Autodesk Inventor part; units mm, degrees
ref_plane "YZ Plane" through (0, 0, 0) normal (1, 0, 0) x (0, 1, 0)
ref_plane "XZ Plane" through (0, 0, 0) normal (0, 1, 0) x (-1, 0, 0)
ref_plane "XY Plane" through (0, 0, 0) normal (0, 0, 1) x (1, 0, 0)
sketch "Skizze1" plane through (0, 0, 0) normal (0, 1, 0) x (-1, 0, 0)
  line L0 (0, 0) -> (62, 0)
  line L1 (62, 0) -> (62, -62)
  line L2 (62, -62) -> (0, -62)
  line L3 (0, -62) -> (0, 0)
  line L4 (2, -2) -> (6, -2)
  line L5 (6, -2) -> (6, -6)
  line L6 (6, -6) -> (2, -6)
  line L7 (2, -6) -> (2, -2)
  line L8 (2, -56) -> (6, -56)
  line L9 (6, -56) -> (6, -60)
  line L10 (6, -60) -> (2, -60)
  line L11 (2, -60) -> (2, -56)
  line L12 (56, -2) -> (60, -2)
  line L13 (60, -2) -> (60, -6)
  line L14 (60, -6) -> (56, -6)
  line L15 (56, -6) -> (56, -2)
  line L16 (56, -56) -> (60, -56)
  line L17 (60, -56) -> (60, -60)
  line L18 (60, -60) -> (56, -60)
  line L19 (56, -60) -> (56, -56)
  line L20 (3, -3) -> (59, -3)
  line L21 (59, -3) -> (59, -59)
  line L22 (59, -59) -> (3, -59)
  line L23 (3, -59) -> (3, -3)
  point P0 (2, -58)
  point P1 (6, -3)
  point P2 (56, -3)
  point P3 (59, -6)
  point P4 (59, -56)
  point P5 (56, -59)
  point P6 (6, -59)
  point P7 (3, -56)
  point P8 (3, -6)
  dimension "d0" = 62
  dimension "d1" = 62
  dimension "d2" = 4
  dimension "d3" = 4
  dimension "d4" = 4
  dimension "d5" = 4
  dimension "d6" = 4
  dimension "d7" = 50
  dimension "d8" = 50
  dimension "d9" = 2
  dimension "d10" = 2
  dimension "d11" = 2
  dimension "d12" = 56
  dimension "d13" = 56
extrude "Extrusion1" add sketch "Skizze1" along normal blind 4
sketch "Skizze2" plane through (0, 4, 0) normal (0, 1, 0) x (1, 0, 0)
  line L0 (-2, 2) -> (-6, 2)
  line L1 (-3, 6) -> (-2, 6)
  line L2 (-6, 2) -> (-2, 2)
  line L3 (-2, 2) -> (-2, 6)
  line L4 (-2, 6) -> (-6, 6)
  line L5 (-6, 6) -> (-6, 2)
  line L6 (-62, 0) -> (0, 0)
  line L7 (0, 0) -> (0, 62)
  line L8 (-6, 0) -> (0, 0)
  line L9 (0, 0) -> (0, 6)
  line L10 (0, 6) -> (-6, 6)
  line L11 (-6, 6) -> (-6, 0)
  line L12 (0, 62) -> (-62, 62)
  line L13 (0, 55.9421) -> (-6, 55.9421)
  line L14 (-6, 55.9421) -> (-6, 62)
  line L15 (-6, 62) -> (0, 62)
  line L16 (0, 62) -> (0, 55.9421)
  line L17 (-6, 59) -> (-6, 60)
  line L18 (-6, 60) -> (-2, 60)
  line L19 (-2, 60) -> (-2, 56)
  line L20 (-2, 56) -> (-6, 56)
  line L21 (-6, 56) -> (-6, 60)
  line L22 (-62, 62) -> (-56, 62)
  line L23 (-56, 62) -> (-56, 55.9421)
  line L24 (-56, 55.9421) -> (-62, 55.9421)
  line L25 (-62, 55.9421) -> (-62, 62)
  line L26 (-60, 60) -> (-56, 60)
  line L27 (-60, 60) -> (-56, 60)
  line L28 (-56, 60) -> (-56, 55.9421)
  line L29 (-56, 55.9421) -> (-60, 55.9421)
  line L30 (-60, 55.9421) -> (-60, 60)
  line L31 (-62, 62) -> (-62, 0)
  line L32 (-62, 6) -> (-56, 6)
  line L33 (-56, 6) -> (-56, 0)
  line L34 (-56, 0) -> (-62, 0)
  line L35 (-62, 0) -> (-62, 6)
  line L36 (-56, 2) -> (-60, 2)
  line L37 (-60, 2) -> (-60, 6)
  line L38 (-60, 6) -> (-56, 6)
  line L39 (-56, 6) -> (-56, 2)
extrude "Extrusion2" add sketch "Skizze2" along normal blind 25 contours L3 L10 L7 L6 L11 L0 | L6 L31 L32 L37 L36 L33 | L13 L14 L20 L19 L18 L12 L7 | L25 L12 L23 L26 L30 L24
sketch "Skizze3" plane through (0, 29, 0) normal (0, 1, 0) x (1, 0, 0)
  line L0 (-62, 0) -> (0, 0)
  line L1 (0, 0) -> (-62, 0)
  line L2 (-62, 0) -> (-62, 62)
  line L3 (-62, 62) -> (0, 62)
  line L4 (0, 62) -> (0, 0)
  line L5 (-6, 6) -> (-56, 6)
  line L6 (-56, 6) -> (-56, 56)
  line L7 (-56, 56) -> (-6, 56)
  line L8 (-6, 56) -> (-6, 6)
  line L9 (-60, 2) -> (-60, 6)
  line L10 (-56, 6) -> (-60, 6)
  line L11 (-60, 6) -> (-60, 2)
  line L12 (-60, 2) -> (-56, 2)
  line L13 (-56, 2) -> (-56, 6)
  line L14 (-60, 60) -> (-56, 60)
  line L15 (-56, 56) -> (-60, 56)
  line L16 (-60, 56) -> (-60, 60)
  line L17 (-60, 60) -> (-56, 60)
  line L18 (-56, 60) -> (-56, 56)
  line L19 (-3, 56) -> (-6, 56)
  line L20 (-2, 60) -> (-2, 56)
  line L21 (-6, 56) -> (-2, 56)
  line L22 (-2, 56) -> (-2, 60)
  line L23 (-2, 60) -> (-6, 60)
  line L24 (-6, 60) -> (-6, 56)
  line L25 (-2, 2) -> (-6, 2)
  line L26 (-6, 6) -> (-2, 6)
  line L27 (-2, 6) -> (-2, 2)
  line L28 (-2, 2) -> (-6, 2)
  line L29 (-6, 2) -> (-6, 6)
  dimension "d18" = 50
  dimension "d19" = 50
extrude "Extrusion3" add sketch "Skizze3" along normal blind 4
sketch "Skizze4" plane through (0, 29, 0) normal (0, -1, 0) x (1, 0, 0)
  line L0 (-6, -6) -> (-56, -6)
  line L1 (-6, -6) -> (-2, -6)
  line L2 (-2, -6) -> (-2, -56)
  line L3 (-2, -56) -> (-6, -56)
  line L4 (-6, -56) -> (-6, -6)
  line L5 (-6, -56) -> (-56, -56)
  line L6 (-56, -56) -> (-56, -60)
  line L7 (-56, -60) -> (-6, -60)
  line L8 (-6, -60) -> (-6, -56)
  line L9 (-56, -6) -> (-56, -2)
  line L10 (-56, -6) -> (-6, -6)
  line L11 (-6, -6) -> (-6, -2)
  line L12 (-6, -2) -> (-56, -2)
  line L13 (-56, -2) -> (-56, -6)
  line L14 (-60, -6) -> (-56, -6)
  line L15 (-56, -6) -> (-60, -6)
  line L16 (-60, -6) -> (-60, -56)
  line L17 (-60, -56) -> (-56, -56)
  line L18 (-56, -56) -> (-56, -6)
  point P0 (0, 0)
  dimension "d22" = 4
  dimension "d23" = 50
  dimension "d24" = 50
  dimension "d25" = 4
  dimension "d26" = 50
  dimension "d27" = 4
  dimension "d28" = 4
  dimension "d29" = 50
extrude "Extrusion4" cut sketch "Skizze4" against normal blind 2 contours L1 L2 L3 L4 | L0 L9 L12 L11 | L18 L17 L16 L14 | L8 L7 L6 L5
sketch "Skizze5" plane through (0, 31, 0) normal (0, -1, 0) x (1, 0, 0)
  line L0 (-59, -59) -> (-3, -59)
  line L1 (-3, -59) -> (-3, -3)
  line L2 (-59, -3) -> (-59, -59)
  line L3 (-57.5, -4.5) -> (-57.5, -57.5)
  line L4 (-57.5, -57.5) -> (-4.5, -57.5)
  line L5 (-4.5, -57.5) -> (-4.5, -4.5)
  line L6 (-62, 0) -> (0, 0)
  line L7 (0, 0) -> (0, -62)
  line L8 (-60, -60) -> (-56, -60)
  line L9 (-2, -6) -> (-2, -2)
  line L10 (-60, -60) -> (-2, -60)
  line L11 (-2, -60) -> (-2, -2)
  line L12 (-2, -2) -> (-60, -2)
  line L13 (-60, -2) -> (-60, -60)
  dimension "d32" = 56
  dimension "d33" = 56
  dimension "d34" = 53
  dimension "d35" = 53
  dimension "d36" = 1.5
  dimension "d39" = 3
extrude "Extrusion5" cut sketch "Skizze5" against normal blind 1
sketch "Skizze6" plane through (0, 32, 0) normal (0, -1, 0) x (1, 0, 0)
  line L0 (-60, -6) -> (-56, -6)
  line L1 (-56, -6) -> (-52, -6)
  line L2 (-6, -6) -> (-56, -6)
  line L3 (-52, -6) -> (-56, -10)
  line L4 (-56, -6) -> (-56, -56)
  line L5 (-56, -10) -> (-56, -6)
  line L6 (-6, -56) -> (-6, -6)
  line L7 (-6, -6) -> (-10, -6)
  line L8 (-6, -6) -> (-2, -6) construction
  line L9 (-10, -6) -> (-6, -10)
  line L10 (-6, -10) -> (-6, -6)
  line L11 (-6, -56) -> (-6, -60)
  line L12 (-6, -56) -> (-6, -52)
  line L13 (-6, -52) -> (-10, -56)
  line L14 (-56, -56) -> (-6, -56)
  line L15 (-56, -56) -> (-52, -56)
  line L16 (-56, -52) -> (-52, -56)
  line L17 (-56, -52) -> (-56, -56)
  point P0 (0, 0)
  dimension "d42" = 4
  dimension "d43" = 45
  dimension "d44" = 4
  dimension "d45" = 180
extrude "Extrusion6" add sketch "Skizze6" against normal blind 1 contours L1 L3 L4 | L2 L6 L9 | L16 L14 L4 | L6 L14 L13
sketch "Skizze7" plane through (-6, 4, -55.9421) normal (0, 0, 1) x (1, 0, 0)
  line L0 (3, 0) -> (0, 0)
  line L1 (0, 0) -> (4, 0)
  line L2 (4, 0) -> (4, 25)
  line L3 (4, 25) -> (0, 25)
  line L4 (0, 25) -> (0, 0)
  point P0 (6, -4)
extrude "Extrusion7" cut sketch "Skizze7" against normal blind 1
sketch "Skizze10" plane through (0, 29, 0) normal (0, -1, 0) x (1, 0, 0)
  line L0 (-2, -6) -> (-2, -55.9421)
  line L1 (-6, -6) -> (-2, -6)
  line L2 (-2, -6) -> (-6, -6)
  line L3 (-6, -2) -> (-6, -6)
  line L4 (-6, -6) -> (-6, -2)
  line L5 (-56, -3) -> (-56, -2)
  line L6 (-6, -2) -> (-56, -2)
  line L7 (-56, -6) -> (-56, -2)
  line L8 (-56, -2) -> (-56, -6)
  line L9 (-60, -6) -> (-56, -6)
  line L10 (-56, -6) -> (-60, -6)
  line L11 (-60, -56) -> (-60, -60)
  line L12 (-60, -6) -> (-60, -56)
  line L13 (-56, -56) -> (-60, -56)
  line L14 (-60, -56) -> (-56, -56)
  line L15 (-56, -60) -> (-56, -56)
  line L16 (-56, -56) -> (-56, -60)
  line L17 (-6, -59) -> (-6, -60)
  line L18 (-56, -60) -> (-6, -60)
  line L19 (-6, -56) -> (-6, -60)
  line L20 (-6, -60) -> (-6, -56)
  line L21 (-3, -56) -> (-2, -56)
  line L22 (-6, -56) -> (-2, -56)
  line L23 (-2, -56) -> (-2, -6)
  line L24 (0, -6) -> (0, -55.9421)
  line L25 (-2, -6) -> (0, -6)
  line L26 (0, -6) -> (0, -56)
  line L27 (0, -56) -> (-2, -56)
  line L28 (-6, -62) -> (-56, -62)
  line L29 (-6, -60) -> (-6, -62)
  line L30 (-6, -62) -> (-56, -62)
  line L31 (-56, -62) -> (-56, -60)
  line L32 (-56, 0) -> (-6, 0)
  line L33 (-56, -2) -> (-56, 0)
  line L34 (-56, 0) -> (-6, 0)
  line L35 (-6, -2) -> (-6, 0)
  line L36 (-6, 0) -> (-6, -2)
  line L37 (-60, -6) -> (-62, -6)
  line L38 (-62, -62) -> (-62, 0)
  line L39 (-62, -56) -> (-62, -6)
  line L40 (-59, -6) -> (-59, -56)
  line L41 (-62, -56) -> (-60, -56)
  point P0 (0, 0)
extrude "Extrusion8" add sketch "Skizze10" along normal blind 1
sketch "Skizze11" plane through (0, 0, 0) normal (0, -1, 0) x (1, 0, 0)
  line L0 (-60, -60) -> (-56, -60)
  line L1 (-2, -6) -> (-2, -2)
  line L2 (-60, -60) -> (-2, -60)
  line L3 (-2, -60) -> (-2, -2)
  line L4 (-2, -2) -> (-60, -2)
  line L5 (-60, -2) -> (-60, -60)
  line L6 (-1, -1) -> (-61, -1)
  line L7 (-61, -1) -> (-61, -61)
  line L8 (-61, -61) -> (-1, -61)
  line L9 (-1, -61) -> (-1, -1)
  point P0 (0, 0)
  dimension "d52" = 60
  dimension "d53" = 60
extrude "Extrusion9" add sketch "Skizze11" against normal blind 28
sketch "Skizze13" plane through (-56, 28, -1) normal (0, 0, 1) x (1, 0, 0)
  line L0 (0, -24) -> (50, -24)
  line L1 (0, 0) -> (-4, 0)
  line L2 (50, -24) -> (0, -24)
  line L3 (0, -24) -> (0, 0)
  line L4 (0, 0) -> (50, 0)
  line L5 (50, 0) -> (50, -24)
  point P0 (56, -28)
extrude "Extrusion10" cut sketch "Skizze13" against normal blind 1
sketch "Skizze16" plane through (-1, 4, -55.9421) normal (1, 0, 0) x (0, 0, -1)
  line L0 (0, 24) -> (0, 0)
  line L1 (-49.9421, 0) -> (-49.9421, 24)
  line L2 (0, 16.5) -> (-49.9421, 16.5)
  line L3 (-49.9421, 16.5) -> (-49.9421, 14.5)
  line L4 (-49.9421, 14.5) -> (0, 14.5)
  line L5 (0, 14.5) -> (0, 16.5)
  point P0 (-55.9421, -4)
  point P1 (-49.9421, 16.5)
  dimension "d67" = 2
extrude "Extrusion13" cut sketch "Skizze16" against normal blind 5
sketch "Skizze18" plane through (-62, 0, 0) normal (0, 0, 1) x (1, 0, 0)
  line L0 (2, 28) -> (6, 28)
  line L1 (2, 28) -> (22, 28)
  line L2 (2, 28) -> (22, 28) construction
  line L3 (22, 28) -> (22, 26)
  line L4 (56, 28) -> (60, 28)
  line L5 (60, 28) -> (40, 28)
  line L6 (6, 28) -> (56, 28)
  line L7 (40, 28) -> (40, 26)
  line L8 (61, 20.5) -> (60, 20.5)
  line L9 (40, 26) -> (60, 20.5)
  line L10 (60, 20.5) -> (60, 28)
  line L11 (22, 26) -> (2, 20.5)
  line L12 (2, 0) -> (2, 33)
  line L13 (2, 28) -> (2, 20.5)
  point P0 (62, 0)
  dimension "d71" = 20
  dimension "d72" = 0
  dimension "d73" = 2
  dimension "d74" = 20
extrude "Extrusion14" add sketch "Skizze18" against normal blind 60
sketch "Skizze19" plane through (-62, 0, 0) normal (0, 0, 1) x (1, 0, 0)
  line L0 (56, 23.3797) -> (56, 33)
  line L1 (0, 33) -> (62, 33)
  line L2 (56, 33) -> (52, 33)
  line L3 (56, 33) -> (41.5, 33)
  line L4 (52, 33) -> (10, 33)
  line L5 (56, 33) -> (70.5, 33) construction
  line L6 (41.5, 33) -> (41.5, 27.3672)
  line L7 (56, 28) -> (6, 28)
  line L8 (41.5, 27.3672) -> (56, 23.3797)
  line L9 (40, 26) -> (56, 21.6)
  line L10 (6, 28) -> (6, 4)
  line L11 (6, 23.3797) -> (6, 33)
  line L12 (10, 33) -> (6, 33)
  line L13 (6, 33) -> (20.5, 33)
  line L14 (20.5, 33) -> (20.5, 27.3672)
  line L15 (20.5, 27.3672) -> (6, 23.3797)
  point P0 (62, 0)
  dimension "d77" = 14.5
  dimension "d78" = 180
  dimension "d79" = 14.5
extrude "Extrusion15" cut sketch "Skizze19" against normal blind 71.1125 contours L8 L6 L7 L0 | L7 L6 L1 L0 | L14 L15 L10 L7 | L7 L11 L1 L14
sketch "Skizze20" plane through (-1, 4, -6) normal (1, 0, 0) x (0, 0, -1)
  line L0 (0, 16.5) -> (49.9421, 16.5)
  line L1 (0, 16.5) -> (10, 16.5)
  line L2 (10, 16.5) -> (10, 12.5)
  line L3 (10, 12.5) -> (0, 12.5)
  line L4 (0, 12.5) -> (0, 16.5)
  point P0 (-6, -4)
  dimension "d82" = 10
  dimension "d83" = 4
extrude "Extrusion16" cut sketch "Skizze20" against normal blind 2
sketch "Skizze21" plane through (0, 33, 0) normal (0, 1, 0) x (1, 0, 0)
  line L0 (-1, 6) -> (-2, 6)
  line L1 (-6, 0) -> (-6, 2)
  line L2 (-2, 6) -> (-6, 6)
  line L3 (-6, 6) -> (-6, 2)
  line L4 (-6, 2) -> (-2, 2)
  line L5 (-2, 2) -> (-2, 6)
  line L6 (-56, 2) -> (-60, 2)
  line L7 (-60, 2) -> (-60, 6)
  line L8 (-60, 6) -> (-56, 6)
  line L9 (-56, 6) -> (-56, 2)
  line L10 (-60, 56) -> (-60, 60)
  line L11 (-60, 60) -> (-56, 60)
  line L12 (-60, 56) -> (-56, 56)
  line L13 (-56, 56) -> (-56, 60)
  line L14 (-56, 60) -> (-60, 60)
  line L15 (-60, 60) -> (-60, 56)
  line L16 (-6, 60) -> (-2, 60)
  line L17 (-6, 56) -> (-2, 56)
  line L18 (-2, 60) -> (-6, 60)
  line L19 (-6, 60) -> (-6, 56)
  line L20 (-6, 56) -> (-2, 56)
  line L21 (-2, 56) -> (-2, 60)
  point P0 (0, 0)
extrude "Extrusion17" cut sketch "Skizze21" against normal blind 20
sketch "Skizze22" plane through (-60, 29, -6) normal (0, 0, 1) x (1, 0, 0)
  line L0 (54, 0) -> (54, -5.6203)
  line L1 (58, 3) -> (58, 4)
  line L2 (54, -5.6203) -> (58, -5.6203)
  line L3 (58, -5.6203) -> (58, 4)
  line L4 (58, 4) -> (54, 4)
  line L5 (54, 4) -> (54, -5.6203)
  line L6 (4, 0) -> (4, -5.6203)
  line L7 (0, -29) -> (0, 4)
  line L8 (4, -5.6203) -> (0, -5.6203)
  line L9 (0, -5.6203) -> (0, 4)
  line L10 (0, 4) -> (4, 4)
  line L11 (4, 4) -> (4, -5.6203)
  point P0 (60, -29)
extrude "Extrusion18" cut sketch "Skizze22" against normal blind 51.4375
properties part number "Unterbau V3"
Here's how the part is built. I have some questions about the finished solid (model axes, mm). A direction names the side the tool comes from. Round coordinates to 2 decimals unless told otherwise and drop trailing zeros. Order: outer loops, then holes, each group sorted by start corner. A loop starts at its lowest first (then second) coordinate and runs counter-clockwise, first axis right, second up. Notation, with made-up numbers: (21.25, 0.5) -> (51.25, 0.5) arc R17 ccw to (51.25, 23.5) -> close; hole circle Ø4 at (70, 42). An arc over 180 degrees is marked (long way). Return JSON: item names as keys, results as strings.
Q1. I need wall thicknesses on line 1 along X through (y, z) = (27.5, -9.5); line 2 along X through (y, z) = (11, -6.5); line 3 along X through (y, z) = (3.5, -30.5). Which ranges of each line are inside material? Lowest first, please. Write a range as from..to.
Filled sheet:
{"line 1": "x = -61..-60, -41.5..-40, -22..-20.5, -2..-1", "line 2": "x = -61..-60, -2..-1", "line 3": "x = -62..-59, -3..0"}
Q2. If we section it at C-C on y = 3: List the corners of the cut face in (x, z) for me.
Filled sheet:
{"outline": "(-62, -62) -> (0, -62) -> (0, 0) -> (-62, 0) -> close; hole (-60, -60) -> (-56, -60) -> (-56, -59) -> (-6, -59) -> (-6, -60) -> (-2, -60) -> (-2, -56) -> (-3, -56) -> (-3, -6) -> (-2, -6) -> (-2, -2) -> (-6, -2) -> (-6, -3) -> (-56, -3) -> (-56, -2) -> (-60, -2) -> (-60, -6) -> (-59, -6) -> (-59, -56) -> (-60, -56) -> close"}
Q3. If we section it at D-D on y = 7.5: List the corners of the cut face in (x, z) for me.
Filled sheet:
{"outline": "(-62, -62) -> (-56, -62) -> (-56, -61) -> (-6, -61) -> (-6, -62) -> (0, -62) -> (0, -55.94) -> (-1, -55.94) -> (-1, -6) -> (0, -6) -> (0, 0) -> (-6, 0) -> (-6, -2) -> (-2, -2) -> (-2, -60) -> (-60, -60) -> (-60, -2) -> (-56, -2) -> (-56, 0) -> (-62, 0) -> (-62, -6) -> (-61, -6) -> (-61, -55.94) -> (-62, -55.94) -> close"}
Q4. If we section it at B-B on z = -57.5: List the corners of the cut face in (x, y) for me.
Filled sheet:
{"outline": "(-62, 0) -> (-60, 0) -> (-60, 33) -> (-62, 33) -> close; (-56, 21.6) -> (-40, 26) -> (-40, 28) -> (-22, 28) -> (-22, 26) -> (-6, 21.6) -> (-6, 23.38) -> (-20.5, 27.37) -> (-20.5, 29) -> (-41.5, 29) -> (-41.5, 27.37) -> (-56, 23.38) -> close; (-41.5, 32) -> (-20.5, 32) -> (-20.5, 33) -> (-41.5, 33) -> close; (-2, 0) -> (0, 0) -> (0, 33) -> (-2, 33) -> close"}
Q5. If we mould it in two halves opening along Y, with no side actions, what happens to faces 4 (the flat face through (-31, 33, -59)), 5 (the flat face through (-29, 0, -61)), 6 (the flat face through (-0.5, 15.8, -6))? For each: released by +Y, released by -Y, zero draft, split by the parting line, or undercut.
Filled sheet:
{"face 4": "released by +Y", "face 5": "released by -Y", "face 6": "undercut"}
Q6. For pin 1 Ø0.8 at (x, z) = (-28.5, -61.5) entering from -Y; pin 2 Ø1.5 at (x, z) = (-47.5, -25.5) entering from +Y; pin 3 Ø3 at (x, y) = (-31.5, 15.5) entering from +Z; pin 4 Ø3 at (x, y) = (-28, 12.5) entering from -Z, each with a flat end and sliding along its axis, tell me the tip position at first contact or that it passes through.
Filled sheet:
{"pin 1": "stops at y = 0", "pin 2": "stops at y = 25.92", "pin 3": "stops at z = -60", "pin 4": "stops at z = -61"}
Q7. If we section it at A-A on x = -33: List the corners of the cut face in (y, z) for me.
Filled sheet:
{"outline": "(0, -62) -> (4, -62) -> (4, -61) -> (28, -61) -> (28, -62) -> (33, -62) -> (33, -56) -> (32, -56) -> (32, -60) -> (29, -60) -> (29, -2) -> (32, -2) -> (32, -6) -> (33, -6) -> (33, 0) -> (28, 0) -> (28, -60) -> (4, -60) -> (4, -59) -> (0, -59) -> close; (0, -3) -> (4, -3) -> (4, 0) -> (0, 0) -> close"}
Q8. Which directions (+Z, -Z, +X, -X, +Y, -Y) give clear straight access to the entire face, cutting with the end or side of a thin tool? Please do faces 1 (the flat face through (-31, 16, -61)), 2 (the flat face through (-31, 29, -31)), 3 (the flat face through (-0.5, 16.2, -55.942)).
Filled sheet:
{"face 1": "-Z", "face 2": "none", "face 3": "+X"}
